Drawing for the job (mm, zero at the part's lowest x, y, z). A direction names the side the tool comes from. Give positions to 0.01 mm unless a question says otherwise; leave off trailing zeros. Write each loop counter-clockwise with the first axis right and the second up, starting at its lowest first coordinate (ties: lowest second). Pieces come first, ordered by that corner, then holes. Notation, with made-up numbers: (39.25, 36) - (65.25, 36) arc R30 cw to (65.25, 67) - close; hole circle Ø4 at (-40, -29). An arc over 180 degrees is marked (long way). Use CSV: the item, a comma, the result in double quotes.
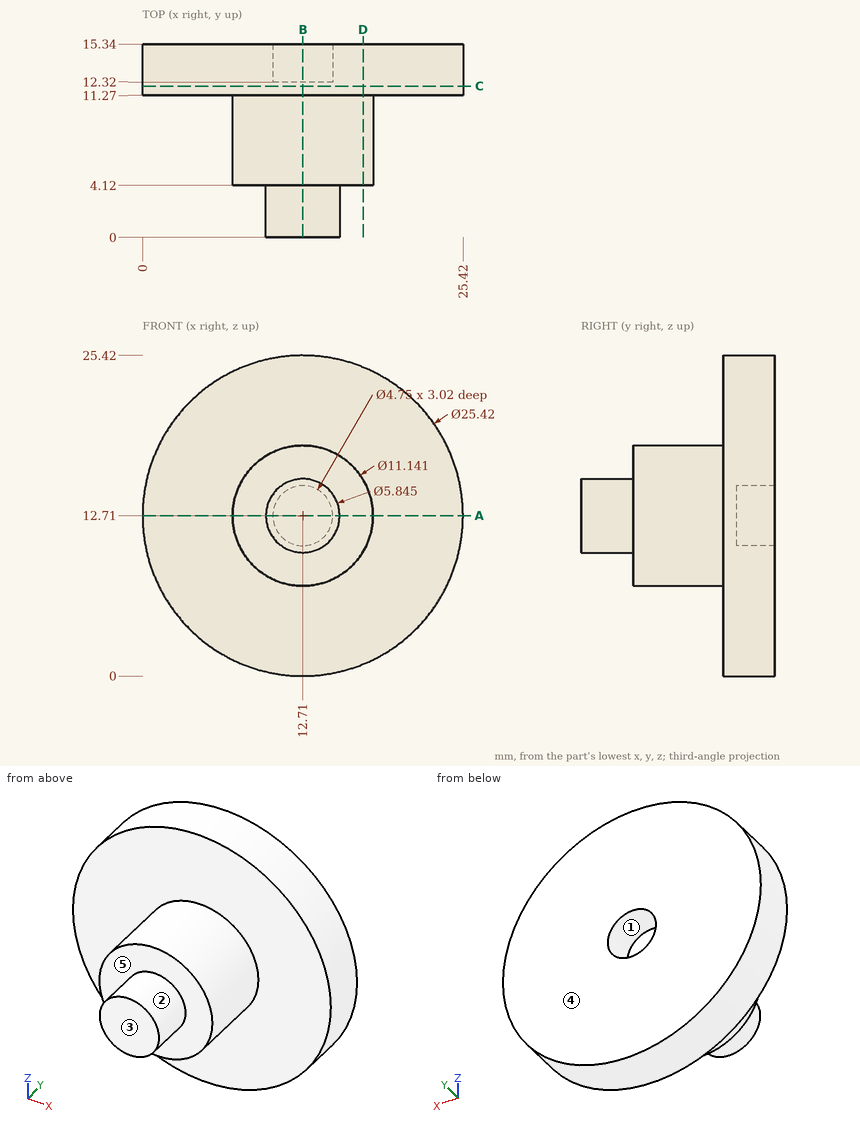
(1) Pull direction Z, two halves, no side cores. Call the marked faces 1, 2 and 3: released by +Z, released by -Z, zero draft, split by the parting line, or undercut.
Checked values:
face 1,"undercut"
face 2,"split by the parting line"
face 3,"zero draft"
(2) Flat gauge pins, fed straight in: P1, Ø1.5, axis at y = 13, z = 7, coming from the -X side; P2, Ø10, axis at x = 20, z = 19.5, coming from the -Y side; P3, Ø5, axis at y = 6.5, z = 20, coming from the -X side (1 decimal). Where does each tip first touch, or does it go through?
Checked values:
P1,"stops at x = 1.01"
P2,"stops at y = 4.12"
P3,"stops at x = 9.9"
(3) 3-axis set-ups, long thin cutter, end or side, ignore diameter. For the marked faces 4 and 5: which of +Z, -Z, +X, -X, +Y, -Y reach the whole face in a straight line?
Checked values:
face 4,"+Z, -Z, +X, -X, +Y"
face 5,"-Y"
(4) Saw through at D-D, the plane x = 17.5. List the corners of the cut face in (y, z).
Checked values:
outline,"(4.12, 9.87) - (11.27, 9.87) - (11.27, 0.94) - (15.34, 0.94) - (15.34, 24.48) - (11.27, 24.48) - (11.27, 15.55) - (4.12, 15.55) - close"
(5) Saw through at A-A, the plane z = 12.71. List the corners of the cut face in (x, y) (1 decimal), then the cut area to 3 significant figures.
Checked values:
outline,"(0, 11.3) - (7.1, 11.3) - (7.1, 4.1) - (9.8, 4.1) - (9.8, 0) - (15.6, 0) - (15.6, 4.1) - (18.3, 4.1) - (18.3, 11.3) - (25.4, 11.3) - (25.4, 15.3) - (15.1, 15.3) - (15.1, 12.3) - (10.3, 12.3) - (10.3, 15.3) - (0, 15.3) - close"
area,"193 mm^2"
(6) Saw through at B-B, the plane x = 12.71. List the corners of the cut face in (y, z) (1 decimal), then the cut area to 3 significant figures.
Checked values:
outline,"(0, 9.8) - (4.1, 9.8) - (4.1, 7.1) - (11.3, 7.1) - (11.3, 0) - (15.3, 0) - (15.3, 10.3) - (12.3, 10.3) - (12.3, 15.1) - (15.3, 15.1) - (15.3, 25.4) - (11.3, 25.4) - (11.3, 18.3) - (4.1, 18.3) - (4.1, 15.6) - (0, 15.6) - close"
area,"193 mm^2"
(7) Wall check: probe 1 along Z at (x, y) = (12.71, 13) (1 decimal); probe 2 along Z at (x, y) = (17.75, 4.5) (1 decimal); probe 3 along Y at (x, z) = (9, 18). Give the ranges that are in metal, low to high. Write a range as [from, to].
Checked values:
probe 1,"z = [0, 10.3], [15.1, 25.4]"
probe 2,"z = [10.3, 15.1]"
probe 3,"y = [11.27, 15.34]"
(8) Saw through at C-C, the plane y = 12. List the corners of the cut face in (x, z).
Checked values:
outline,"circle Ø25.42 at (12.71, 12.71)"
